The listing builds one solid part. Answer for the finished solid, in the listing's coordinates (mm). Face numbers are marked on the shaded views. A direction names the side the tool comes from. Coordinates: 2 decimals unless noted, no trailing zeros. Write each loop counter-clockwise with the first axis right and the second up, starting at its lowest first coordinate (ties: lowest second). Pieces come first, ordered by that corner, then holes.
(1) The part is cut by section B-B on x = 2.25. Determine the outline of the cut face in (y, z).
(2) The part is cut by section A-A on z = -7. Determine the outline of the cut face in (x, y), plus the area to 3 significant figures.
(3) Straight lines are drawn through the part: line 1 (Y direction, x = 8.75, z = 1.5); line 2 (Z direction, x = 9, y = 33); line 3 (Z direction, x = -0.75, y = 19.5). For each, find the intervals that lie inside material, in ascending order.
(4) The part is cut by section C-C on y = 36. Determine the outline of the cut face in (x, z), plus the area to 3 significant figures.
(5) Given P1, Ø8, axis at x = 13, y = 27.5, coming from the +Z side; P2, Ø3, axis at x = 3, z = -4, coming from the -Y side; P3, Ø12, axis at y = 39, z = -5, coming from the -X side; P4, Ø10, axis at y = 37.5, z = -11.5, coming from the -X side, each flat-ended and moving along its own axis, determine where each tip first touches the part or whether it passes through.
(6) The part is cut by section D-D on z = 7.25. Determine the outline of the cut face in (x, y), plus the area to 3 significant figures.
(7) For a pull along Y with two mould halves and no side action, classify the marked faces 3, 4, 5 and 6 as +Y half, -Y half, draft (parallel to the pull), parting line (faces both ways), or undercut.
(8) Which of the six approach directions +Z, -Z, +X, -X, +Y, -Y give full straight-line access (tool end or side, diameter ignored) to the marked faces 1 and 2?
from build123d import *

# Parameters (mm, degrees)
EXTRUDE_2_DEPTH = 10
EXTRUDE_3_DEPTH = 3


with BuildPart() as part:
    # 草图2 → 凸台-拉伸2 (new body)
    with BuildSketch(Plane(origin=(0, 0, 0), x_dir=(0, 0, -1), z_dir=(1, 0, 0))):
        Polygon((-15.350951503, 50.748946778), (14.649048497, 50.748946778), (14.649048497, 20.748946778), (11.649048497, 20.748946778), (11.649048497, 47.75022668), (-15.350951503, 47.75022668), align=None)
    extrude(amount=EXTRUDE_2_DEPTH)

    # 草图4 → 凸台-拉伸3 (add)
    with BuildSketch(Plane.XZ.offset(-20.748946778)):
        Polygon((10, -14.649048497), (-10, -14.649048497), (-10, -4.649048497), (10, -4.649048497), (20, -4.649048497), (20, -14.649048497), align=None)
    extrude(amount=EXTRUDE_3_DEPTH)


solid = part.part
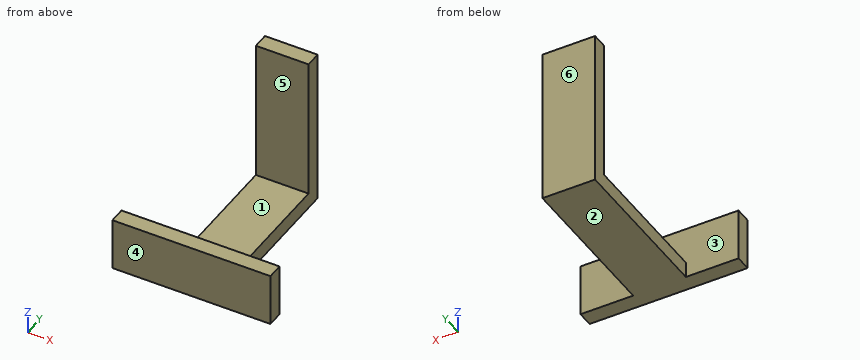
Model answer:
1. outline: (17.75, -14.65) - (50.75, -14.65) - (50.75, 15.35) - (47.75, 15.35) - (47.75, -11.65) - (20.75, -11.65) - (20.75, -4.65) - (17.75, -4.65) - close
2. outline: (-10, 17.75) - (20, 17.75) - (20, 20.75) - (-10, 20.75) - close; (0, 47.75) - (10, 47.75) - (10, 50.75) - (0, 50.75) - close
2. area: 120 mm2
3. line 1: y = 47.75 to 50.75
3. line 2: z = -14.65 to -11.65
3. line 3: z = -14.65 to -4.65
4. outline: (0, -14.65) - (10, -14.65) - (10, -11.65) - (0, -11.65) - close
4. area: 30.0 mm2
5. P1: stops at z = -11.65
5. P2: stops at y = 17.75
5. P3: passes through
5. P4: stops at x = 0
6. outline: (0, 47.75) - (10, 47.75) - (10, 50.75) - (0, 50.75) - close
6. area: 30.0 mm2
7. face 3: undercut
7. face 4: -Y half
7. face 5: undercut
7. face 6: +Y half
8. face 1: +Z, +X, -X
8. face 2: -Z, +X, -X, +Y, -Y
